Design review of the part shown in the three views and the two pictorial views. Dimensions are in mm from the part's minimum x, y and z. A direction names the side the tool comes from. Round coordinates to 2 decimals unless told otherwise and drop trailing zeros. Order: outer loops, then holes, each group sorted by start corner. A loop starts at its lowest first (then second) coordinate and runs counter-clockwise, first axis right, second up.
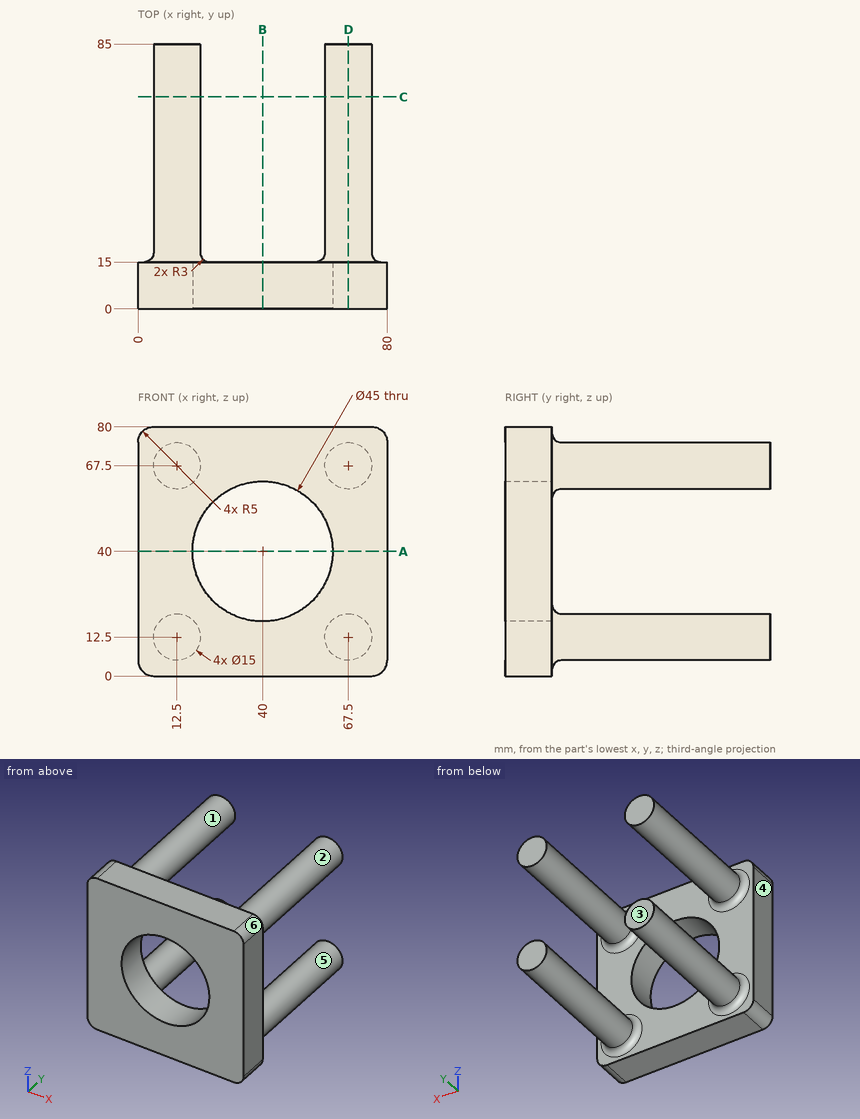
(1) Add section D-D on x = 67.5. Give the boundary of the cut face in (y, z), plus the area to 3 significant figures.
(2) Add section A-A on z = 40. Give the boundary of the cut face in (x, y).
(3) Add section C-C on y = 68. Give the boundary of the cut face in (x, z).
(4) Clearance check with flat-ended pins moving along their axes: P1, Ø1.5, axis at y = 21, z = 72, coming from the +X side; P2, Ø1, axis at y = 56.5, z = 66, coming from the -X side; P3, Ø5, axis at y = 59, z = 16.5, coming from the +X side. State where each tip first meets the part, or that it passes through.
(5) Draft analysis for pull direction X (two halves, no side actions). For the marked faces 1, 2, 3 and 4, state which applies: pulls with the +X half, pulls with the -X half, needs draft (parallel to the pull), parting line crosses it, or undercut.
(6) Tool access review of the marked faces 5 and 6: name each direction out of +Z, -Z, +X, -X, +Y, -Y from which nothing blocks a thin tool from reaching the whole face with its end or side.
(7) Add section B-B on x = 40. Give the boundary of the cut face in (y, z).
(8) Wall thickness on L1, parallel to X at y = 5.75, z = 40; L2, parallel to Y at x = 9, z = 27; L3, parallel to X at y = 67.5, z = 15: over which ranges is each line inside the solid? List them lowest first.
Here are the results:
1. outline: (0, 0) - (15, 0) - (15, 2) arc R3 cw to (18, 5) - (85, 5) - (85, 20) - (18, 20) arc R3 cw to (15, 23) - (15, 57) arc R3 cw to (18, 60) - (85, 60) - (85, 75) - (18, 75) arc R3 cw to (15, 78) - (15, 80) - (0, 80) - close
1. area: 3,310 mm2
2. outline: (0, 0) - (17.5, 0) - (17.5, 15) - (0, 15) - close; (62.5, 0) - (80, 0) - (80, 15) - (62.5, 15) - close
3. outline: circle Ø15 at (12.5, 12.5); circle Ø15 at (12.5, 67.5); circle Ø15 at (67.5, 12.5); circle Ø15 at (67.5, 67.5)
4. P1: stops at x = 74
4. P2: stops at x = 5.07
4. P3: stops at x = 74.85
5. face 1: undercut
5. face 2: undercut
5. face 3: needs draft
5. face 4: pulls with the -X half
6. face 5: +Y
6. face 6: +Z, +X, +Y, -Y
7. outline: (0, 0) - (15, 0) - (15, 17.5) - (0, 17.5) - close; (0, 62.5) - (15, 62.5) - (15, 80) - (0, 80) - close
8. L1: x = 0 to 17.5, 62.5 to 80
8. L2: y = 0 to 15
8. L3: x = 5.43 to 19.57, 60.43 to 74.57
